Check sheet for the drawn part. Datum: minimum x, y, z corner. Units: mm. A direction names the side the tool comes from. Round coordinates to 2 decimals unless told otherwise and drop trailing zeros. Order: outer loops, then holes, each group sorted by start corner. A loop starts at its lowest first (then second) coordinate and runs counter-clockwise, first axis right, second up. Notation, with made-up numbers: (-3.75, -29.75) -> (21.25, -29.75) arc R21 cw to (21.25, -24.75) -> close; hole circle Ø9 at (50, 10). An arc over 180 degrees is marked (long way). Answer in a Markdown table with one row per item.
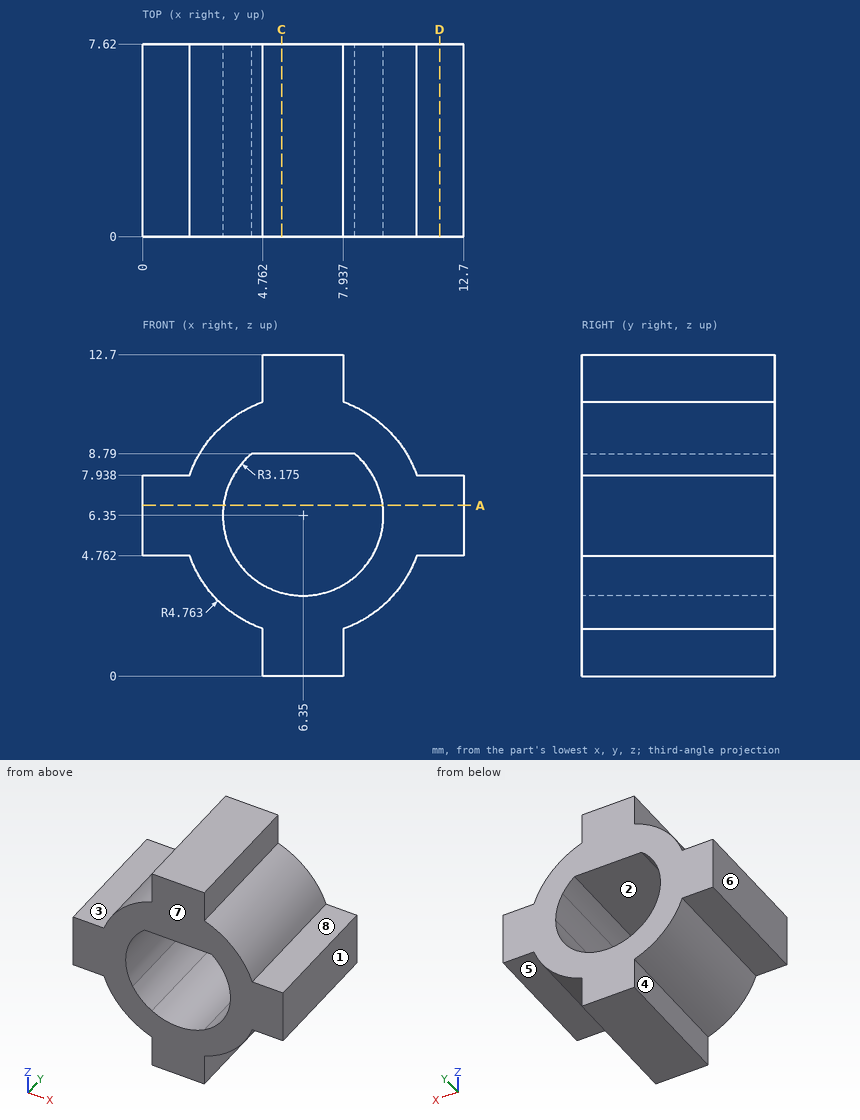
(1) Tool access check on the marked faces 4, 5, 6, 7 and 8. Record the directions out of +Z, -Z, +X, -X, +Y, -Y that give a thin tool (end or side, any length) a straight path to the whole face; none if there is none.
Solutions:
| item | result |
|---|---|
| face 4 | -Z, -X, +Y, -Y |
| face 5 | -Z, +X, +Y, -Y |
| face 6 | +Z, -Z, -X, +Y, -Y |
| face 7 | +Z, -Z, +X, -X, -Y |
| face 8 | +Z, +X, +Y, -Y |
(2) Section check C-C on x = 5.5. Record the boundary of the cut face in (y, z).
Solutions:
| item | result |
|---|---|
| outline | (0, 0) -> (7.62, 0) -> (7.62, 3.29) -> (0, 3.29) -> close; (0, 8.79) -> (7.62, 8.79) -> (7.62, 12.7) -> (0, 12.7) -> close |
(3) Section check A-A on z = 6.75. Record the boundary of the cut face in (x, y).
Solutions:
| item | result |
|---|---|
| outline | (0, 0) -> (3.2, 0) -> (3.2, 7.62) -> (0, 7.62) -> close; (9.5, 0) -> (12.7, 0) -> (12.7, 7.62) -> (9.5, 7.62) -> close |
(4) Depth check by flat-ended pin: pin 1 Ø0.6 at (y, z) = (4, 12) entering from +X; pin 2 Ø0.9 at (x, y) = (11.5, 3) entering from -Z; pin 3 Ø1.5 at (y, z) = (3, 0.5) entering from -X. Enter the tip coordinate at first touch or a pass-through.
Solutions:
| item | result |
|---|---|
| pin 1 | x = 7.94 |
| pin 2 | z = 4.76 |
| pin 3 | x = 4.76 |
(5) Draft check along Z on the marked faces 1, 2 and 3. Enter one of: pulls with the +Z half, pulls with the -Z half, needs draft (parallel to the pull), parting line crosses it, or undercut.
Solutions:
| item | result |
|---|---|
| face 1 | needs draft |
| face 2 | undercut |
| face 3 | pulls with the +Z half |
(6) Section check D-D on x = 11.75. Record the boundary of the cut face in (y, z).
Solutions:
| item | result |
|---|---|
| outline | (0, 4.76) -> (7.62, 4.76) -> (7.62, 7.94) -> (0, 7.94) -> close |
(7) Scan lines: probe 1 along X at (y, z) = (6.75, 11.75); probe 2 along Z at (x, y) = (6, 6.75) (1 decimal); probe 3 along Z at (x, y) = (4.5, 2.25). Record each from-to range of solid material in increasing order. Write a range as from..to.
Solutions:
| item | result |
|---|---|
| probe 1 | 4.76..7.94 |
| probe 2 | 0..3.2, 8.8..12.7 |
| probe 3 | 1.96..3.77, 8.79..10.74 |
